Input: part model. Units: mm. Frame: model coordinates. A direction names the side the tool comes from. Round coordinates to 2 decimals unless told otherwise and drop trailing zeros. Loops run counter-clockwise (first coordinate to the right, second up) from the corner with the lowest first, then second, coordinate; pieces in that order, holes last. Notation, with made-up numbers: (17, -20) -> (37, -20) arc R28 cw to (37, 13) -> close; hole circle Ø3 at (65, 36). An arc over 180 degrees is marked (long way). Answer as a JSON object with one key per item and string values. Group by question number.
Item 1: Set-up query: faces 1 (the flat face through (-75, 0, 50)), 2 (the flat face through (-73, -3, 50)). Return all of +Z, -Z, +X, -X, +Y, -Y with unobstructed straight access to the full face (end or side cutting, diameter ignored); none if empty.
Item 2: Pin query (flat end, axial travel): pin 1 (10 mm diameter, centred on x = -50.5, y = -7.5, fed in from +Z); pin 2 (2.5 mm diameter, centred on x = -146, z = 151.5, fed in from +Y); pin 3 (1 mm diameter, centred on x = -68, z = 111, fed in from -Y); pin 4 (5 mm diameter, centred on y = -26.64, z = 146.81, fed in from -X). Return the tip coordinate at first contact, or that it passes through.
Item 3: Section query B-B on x = -91. Return loops of the section in (y, z).
Item 4: Draft query along Y for faces 3 (the flat face through (-1.479, -37.535, 163.802)), 4 (the flat face through (-52, -2, -44.197)), 5 (the cylindrical face through (-1.52, -28.25, 149.34)). Return one class per face: released by +Y, released by -Y, zero draft, split by the parting line, or undercut.
Item 5: Section query A-A on y = -19.5. Return loops of the section in (x, z), and give its area (3 significant figures).
Item 6: Material intervals for line 1 (X direction, y = -4, z = 59); line 2 (Z direction, x = -2.4, y = -26.64); line 3 (Y direction, x = -61.5, z = -23.5), sorted ascending. Write a range as [from, to].
from build123d import *

# Parameters (mm, degrees)
SKETCH18_W                     = 148
SKETCH18_H                     = 205.5334
BASE_FLANGE1_DEPTH             = 3
EDGE_FLANGE1_STRIP_W           = 13.4732
EDGE_FLANGE1_STRIP_H           = 3
EDGE_FLANGE1_STRIP_CUT_DEPTH   = 205.5334
EDGE_FLANGE1_STRIP_2_W         = 13.4732
EDGE_FLANGE1_STRIP_2_H         = 3
EDGE_FLANGE1_STRIP_CUT_2_DEPTH = 205.5334
EDGE_FLANGE1_DEPTH             = 205.5334
EDGE_FLANGE1_BEND_DEPTH        = 205.5334
SKETCH27_R                     = 3
CUT_EXTRUDE1_DEPTH             = 227.212201998
SKETCH28_W                     = 160
SKETCH28_H                     = 8
CUT_EXTRUDE2_DEPTH             = 25
BOSS_EXTRUDE1_DEPTH            = 5
CHAMFER2_SIZE                  = 5


# Sheet-metal steps are written as plain solids
with BuildPart() as part:
    # Sketch18 → Base-Flange1 (new body)
    with BuildSketch(Plane(origin=(0, 0, 0), x_dir=(1, 0, 0), z_dir=(0, 1, 0))):
        with Locations((-74, -63.57018807)):
            Rectangle(SKETCH18_W, SKETCH18_H)
    extrude(amount=-BASE_FLANGE1_DEPTH)

    # Edge-Flange1 strip (across the edge) → Edge-Flange1 strip cut (cut)
    with BuildSketch(Plane(origin=(0, -3, -39.19651193), x_dir=(-1, 0, 0), z_dir=(0, 0, 1))):
        with Locations((-3, -1.5)):
            Rectangle(EDGE_FLANGE1_STRIP_W, EDGE_FLANGE1_STRIP_H)
    extrude(amount=EDGE_FLANGE1_STRIP_CUT_DEPTH, mode=Mode.SUBTRACT)

    # Edge-Flange1 strip 2 (across the edge) → Edge-Flange1 strip cut 2 (cut)
    with BuildSketch(Plane(origin=(-148, -3, 166.33688807), x_dir=(1, 0, 0), z_dir=(0, 0, -1))):
        with Locations((-3, -1.5)):
            Rectangle(EDGE_FLANGE1_STRIP_2_W, EDGE_FLANGE1_STRIP_2_H)
    extrude(amount=EDGE_FLANGE1_STRIP_CUT_2_DEPTH, mode=Mode.SUBTRACT)

    # Edge-Flange1 section (across the edge) → Edge-Flange1 (add)
    with BuildSketch(Plane(origin=(0, -3, -39.19651193), x_dir=(-1, 0, 0), z_dir=(0, 0, 1))):
        with BuildLine():
            Line((0, 0.7366), (0, 37))
            Line((0, 37), (3, 37))
            Line((3, 37), (3, 0.7366))
            ThreePointArc((3, 0.7366), (3.215745145, 0.215745145), (3.7366, 0))
            Line((3.7366, 0), (3.7366, -3))
            ThreePointArc((3.7366, -3), (1.094424801, -1.905575199), (0, 0.7366))
        make_face()
    extrude(amount=EDGE_FLANGE1_DEPTH)

    # Edge-Flange1 section 2 (across the edge) → Edge-Flange1 bend (add)
    with BuildSketch(Plane(origin=(-148, -3, 166.33688807), x_dir=(1, 0, 0), z_dir=(0, 0, -1))):
        with BuildLine():
            Line((0, 0.7366), (0, 37))
            Line((0, 37), (3, 37))
            Line((3, 37), (3, 0.7366))
            ThreePointArc((3, 0.7366), (3.215745145, 0.215745145), (3.7366, 0))
            Line((3.7366, 0), (3.7366, -3))
            ThreePointArc((3.7366, -3), (1.094424801, -1.905575199), (0, 0.7366))
        make_face()
    extrude(amount=EDGE_FLANGE1_BEND_DEPTH)

    # Sketch27 → Cut-Extrude1 (cut, through all)
    with BuildSketch(Plane.ZY.offset(148)):
        with Locations(Location((-25.19651193, -26.64, 0), (0, 0, 270))):
            Circle(SKETCH27_R)
        with Locations(Location((146.80688807, -26.64, 0), (0, 0, 270))):
            Circle(SKETCH27_R)
    extrude(amount=-CUT_EXTRUDE1_DEPTH, mode=Mode.SUBTRACT)

    # Sketch28 → Cut-Extrude2 (cut)
    with BuildSketch(Plane.XY.offset(166.33688807)):
        with Locations((-79, -2)):
            Rectangle(SKETCH28_W, SKETCH28_H)
    extrude(amount=-CUT_EXTRUDE2_DEPTH, mode=Mode.SUBTRACT)

    # Sketch32 → Boss-Extrude1 (add)
    with BuildSketch(Plane(origin=(0, 0, -39.19651193), x_dir=(-1, 0, 0), z_dir=(0, 0, -1))):
        with BuildLine():
            Line((0, -3.7366), (0, -40))
            Line((0, -40), (3, -40))
            Line((3, -40), (3, -3.7366))
            ThreePointArc((3, -3.7366), (3.215745145, -3.215745145), (3.7366, -3))
            Line((3.7366, -3), (144.2634, -3))
            ThreePointArc((144.2634, -3), (144.784254855, -3.215745145), (145, -3.7366))
            Line((145, -3.7366), (145, -40))
            Line((145, -40), (148, -40))
            Line((148, -40), (148, -3.7366))
            ThreePointArc((148, -3.7366), (146.905575199, -1.094424801), (144.2634, 0))
            Line((144.2634, 0), (3.7366, 0))
            ThreePointArc((3.7366, 0), (1.094424801, -1.094424801), (0, -3.7366))
        make_face()
    extrude(amount=BOSS_EXTRUDE1_DEPTH)

    # Chamfer2
    chamfer2_edges = [part.edges().sort_by_distance(p)[0] for p in [
        (-1.5, -6, 166.33688807),
        (-146.5, -6, 166.33688807),
        (-146.5, -40, -44.19651193),
        (-1.5, -40, -44.19651193),
        (-1.5, -40, 166.33688807),
        (-146.5, -40, 166.33688807),
    ]]
    chamfer(chamfer2_edges, length=CHAMFER2_SIZE)


solid = part.part
Solved:
{
 "1": {"face 1": "+Z, -Z, +X, -X, +Y", "face 2": "+Z, -Z, -Y"},
 "2": {"pin 1": "z = 141.34", "pin 2": "y = -6", "pin 3": "y = -3", "pin 4": "through"},
 "3": {"outline": "(-3, -44.2) -> (0, -44.2) -> (0, 141.34) -> (-3, 141.34) -> close"},
 "4": {"face 3": "released by -Y", "face 4": "zero draft", "face 5": "undercut"},
 "5": {"outline": "(-148, -44.2) -> (-145, -44.2) -> (-145, 166.34) -> (-148, 166.34) -> close; (-3, -44.2) -> (0, -44.2) -> (0, 166.34) -> (-3, 166.34) -> close", "area": "1,260 mm²"},
 "6": {"line 1": "[-148, -145], [-3, 0]", "line 2": "[-44.2, -28.2], [-22.2, 143.81], [149.81, 166.34]", "line 3": "[-3, 0]"}
}
